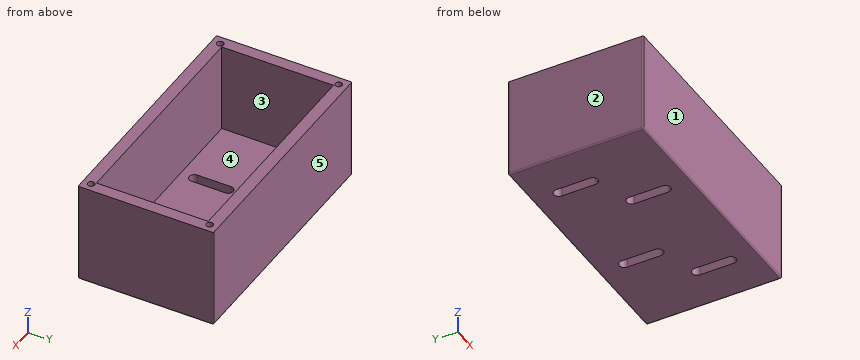
Autodesk Inventor part; units mm, degrees
ref_plane "YZ Plane" through (0, 0, 0) normal (1, 0, 0) x (0, 1, 0)
ref_plane "XZ Plane" through (0, 0, 0) normal (0, 1, 0) x (-1, 0, 0)
ref_plane "XY Plane" through (0, 0, 0) normal (0, 0, 1) x (1, 0, 0)
sketch "Sketch1" plane through (0, 0, 0) normal (0, 0, 1) x (1, 0, 0)
  line L0 (-42.0539, 29.2948) -> (30.7461, 29.2948)
  line L1 (30.7461, 29.2948) -> (30.7461, -10.7052)
  line L2 (30.7461, -10.7052) -> (-42.0539, -10.7052)
  line L3 (-42.0539, -10.7052) -> (-42.0539, 29.2948)
  point P0 (0, 0)
  dimension "d0" = 72.8
  dimension "d1" = 40
extrude "Extrusion1" add sketch "Sketch1" along normal blind 30
shell "Shell2" thickness 3.5 removed faces 1 at (-17.7872, 15.9615, 30)
sketch "Sketch4" plane through (0, 0, 30) normal (0, 0, 1) x (1, 0, 0)
  circle A0 centre (-39.5539, 26.7948) radius 1
  line L0 (30.7461, 29.2948) -> (-42.0539, 29.2948)
  line L1 (-42.0539, 29.2948) -> (-42.0539, -10.7052)
  line L2 (-5.6539, 34.5623) -> (-5.6539, 23.6795)
  circle A1 centre (28.2461, 26.7948) radius 1
  line L3 (36.847, 9.2948) -> (23.7014, 9.2948)
  circle A2 centre (28.2461, -8.2052) radius 1
  circle A3 centre (-39.5539, -8.2052) radius 1
  point P0 (0, 0)
  dimension "d26" = 2
  dimension "d27" = 2.5
  dimension "d28" = 2.5
extrude "Extrusion4" cut sketch "Sketch4" against normal blind 4
fillet "Fillet1" radius 0.4 8 edges at (-42.0539, 29.2948, 15) (-42.0539, -10.7052, 15) (30.7461, -10.7052, 15) (30.7461, 29.2948, 15) (-5.6539, -10.7052, 0) (30.7461, 9.2948, 0) (-5.6539, 29.2948, 0) (-42.0539, 9.2948, 0)
sketch "Sketch5" plane through (0, 0, 0) normal (0, 0, -1) x (-1, 0, 0)
  line L0 (41.6539, -10.7052) -> (-30.3461, -10.7052)
  line L1 (5.6539, -10.7052) -> (5.6539, 29.2948)
  line L2 (-30.3461, 29.2948) -> (41.6539, 29.2948)
  circle A0 centre (22.8539, 9.2948) radius 9.5
  circle A1 centre (-11.5461, 9.2948) radius 9.5
  line L3 (-17.5461, 6.9294) -> (-17.5461, -3.0706) construction
  line L4 (-19.0461, 6.9294) -> (-19.0461, -3.0706)
  line L5 (-16.0461, -3.0706) -> (-16.0461, 6.9294)
  arc A2 (-16.0461, 6.9294) -> (-19.0461, 6.9294) centre (-17.5461, 6.9294) ccw
  arc A3 (-19.0461, -3.0706) -> (-16.0461, -3.0706) centre (-17.5461, -3.0706) ccw
  line L6 (-5.5461, 11.6603) -> (-5.5461, 21.6603) construction
  line L7 (-4.0461, 11.6603) -> (-4.0461, 21.6603)
  line L8 (-7.0461, 21.6603) -> (-7.0461, 11.6603)
  arc A4 (-7.0461, 11.6603) -> (-4.0461, 11.6603) centre (-5.5461, 11.6603) ccw
  arc A5 (-4.0461, 21.6603) -> (-7.0461, 21.6603) centre (-5.5461, 21.6603) ccw
  line L9 (16.8539, 6.9294) -> (16.8539, -3.0706) construction
  line L10 (15.3539, 6.9294) -> (15.3539, -3.0706)
  line L11 (18.3539, -3.0706) -> (18.3539, 6.9294)
  arc A6 (18.3539, 6.9294) -> (15.3539, 6.9294) centre (16.8539, 6.9294) ccw
  arc A7 (15.3539, -3.0706) -> (18.3539, -3.0706) centre (16.8539, -3.0706) ccw
  line L12 (28.8539, 11.6603) -> (28.8539, 21.6603) construction
  line L13 (30.3539, 11.6603) -> (30.3539, 21.6603)
  line L14 (27.3539, 21.6603) -> (27.3539, 11.6603)
  arc A8 (27.3539, 11.6603) -> (30.3539, 11.6603) centre (28.8539, 11.6603) ccw
  arc A9 (30.3539, 21.6603) -> (27.3539, 21.6603) centre (28.8539, 21.6603) ccw
  point P0 (0, 0)
  point P1 (-17.5461, 1.9294)
  point P2 (-5.5461, 16.6603)
  point P3 (16.8539, 1.9294)
  point P4 (28.8539, 16.6603)
  dimension "d32" = 19
  dimension "d33" = 19
  dimension "d34" = 5
  dimension "d35" = 3
  dimension "d36" = 5
  dimension "d37" = 3
  dimension "d38" = 5
  dimension "d39" = 3
  dimension "d40" = 5
  dimension "d41" = 3
  dimension "d42" = 17.2
  dimension "d43" = 17.2
  dimension "d44" = 6
  dimension "d45" = 12
  dimension "d46" = 6
  dimension "d47" = 12
  dimension "d52" = 20
  dimension "d53" = 20
extrude "Extrusion5" cut sketch "Sketch5" against normal through all contours L13 A8 L14 A0 | A0 L14 A9 L13 | L11 A7 L10 A0 | A0 L10 A6 L11 | L7 A4 L8 A1 | A1 L8 A5 L7 | L5 A3 L4 A1 | A1 L4 A2 L5
properties part number "Solenoids_holder"
Geometry: final body of the model. Coordinates: model frame, mm. Face numbers are marked on the shaded views. A direction names the side the tool comes from. Round coordinates to 2 decimals unless told otherwise and drop trailing zeros. Loops run counter-clockwise (first coordinate to the right, second up) from the corner with the lowest first, then second, coordinate; pieces in that order, holes last. Notation, with made-up numbers: (-31.5, 8) -> (-3.5, 8) arc R16 ccw to (-3.5, 30) -> close; hole circle Ø2 at (46.25, -39). An arc over 180 degrees is marked (long way). Use one line per item in the form item = value. Start each with the question number.
1) Section D-D on z = 27.75. Output: boundary loops of the cut face in (x, y).
2) Draft query along X for the marked faces 1, 2 and 3. Return one class per face: released by +X, released by -X, zero draft, split by the parting line, or undercut.
3) Line query: L1, parallel to X at y = 1, z = 3.25; L2, parallel to X at y = -6.5, z = 18.75; L3, parallel to Y at x = 7, z = 22. Output: solid intervals per line, ascending.
4) Section A-A on x = 18. Output: boundary loops of the cut face in (y, z), then the cut area to 3 significant figures.
5) Section B-B on z = 24. Output: boundary loops of the cut face in (x, y), then the cut area to 3 significant figures.
6) Section C-C on y = 17. Output: boundary loops of the cut face in (x, z).
7) Access query for the marked faces 4 and 5. Directions: +Z, -Z, +X, -X, +Y, -Y. A direction counts if a zero-diameter tool reaches every point of the face in a straight line with its end or side. Return the directions, or none.
Response:
q1.outline = (-42.05, -10.31) arc R0.4 ccw to (-41.65, -10.71) -> (30.35, -10.71) arc R0.4 ccw to (30.75, -10.31) -> (30.75, 28.89) arc R0.4 ccw to (30.35, 29.29) -> (-41.65, 29.29) arc R0.4 ccw to (-42.05, 28.89) -> close; hole circle Ø2 at (-39.55, -8.21); hole circle Ø2 at (-39.55, 26.79); hole (-38.55, -7.21) -> (27.25, -7.21) -> (27.25, 25.79) -> (-38.55, 25.79) -> close; hole circle Ø2 at (28.25, -8.21); hole circle Ø2 at (28.25, 26.79)
q2.face_1 = zero draft
q2.face_2 = released by -X
q2.face_3 = undercut
q3.L1 = -42.05 to -18.35, -15.35 to 16.05, 19.05 to 30.75
q3.L2 = -42.05 to -38.55, 27.25 to 30.75
q3.L3 = -10.71 to -7.21, 25.79 to 29.29
q4.outline = (-10.71, 0.4) arc R0.4 ccw to (-10.31, 0) -> (-4.5, 0) -> (-4.5, 3.5) -> (-7.21, 3.5) -> (-7.21, 30) -> (-10.71, 30) -> close; (8.36, 0) -> (28.89, 0) arc R0.4 ccw to (29.29, 0.4) -> (29.29, 30) -> (25.79, 30) -> (25.79, 3.5) -> (8.36, 3.5) -> close
q4.area = 280 mm^2
q5.outline = (-42.05, -10.31) arc R0.4 ccw to (-41.65, -10.71) -> (30.35, -10.71) arc R0.4 ccw to (30.75, -10.31) -> (30.75, 28.89) arc R0.4 ccw to (30.35, 29.29) -> (-41.65, 29.29) arc R0.4 ccw to (-42.05, 28.89) -> close; hole (-38.55, -7.21) -> (27.25, -7.21) -> (27.25, 25.79) -> (-38.55, 25.79) -> close
q5.area = 740 mm^2
q6.outline = (-42.05, 0.4) arc R0.4 ccw to (-41.65, 0) -> (-30.35, 0) -> (-30.35, 3.5) -> (-38.55, 3.5) -> (-38.55, 30) -> (-42.05, 30) -> close; (-27.35, 0) -> (4.05, 0) -> (4.05, 3.5) -> (-27.35, 3.5) -> close; (7.05, 0) -> (30.35, 0) arc R0.4 ccw to (30.75, 0.4) -> (30.75, 30) -> (27.25, 30) -> (27.25, 3.5) -> (7.05, 3.5) -> close
q7.face_4 = +Z
q7.face_5 = +Z, -Z, +X, -X, +Y
